Design review of the part shown in the three views and the two pictorial views. Dimensions are in mm from the part's minimum x, y and z. Give positions to 0.01 mm unless a question says otherwise; leave off trailing zeros. Loops run counter-clockwise (first coordinate to the right, second up) from the corner with the lowest first, then second, coordinate; pieces in that order, holes last. Notation, with made-up numbers: (11.5, 88) -> (19.5, 88) arc R22 cw to (19.5, 113) -> close; hole circle Ø4 at (47.5, -13.75). An arc over 180 degrees is marked (long way). Answer as CSV lines item,"result". Start each with the question number.
Item 1: Add section A-A on x = 112.2. State the section outline as (y, z) points, plus the area to 3 significant figures.
Item 2: Add section B-B on z = 23.5. State the section outline as (x, y) points, plus the area to 3 significant figures.
Item 3: Add section D-D on x = 74. State the section outline as (y, z) points, plus the area to 3 significant figures.
Item 4: For L1, parallel to Z at x = 5, y = 1; L2, parallel to X at y = 1.2, z = 71; L3, parallel to X at y = 0.35, z = 37, list the stretches that pass through material, from the lowest coordinate up. Write a range as from..to.
Item 5: Add section C-C on y = 0.5. State how many separate pieces and enclosed holes the cut face has, plus the area to 3 significant figures.
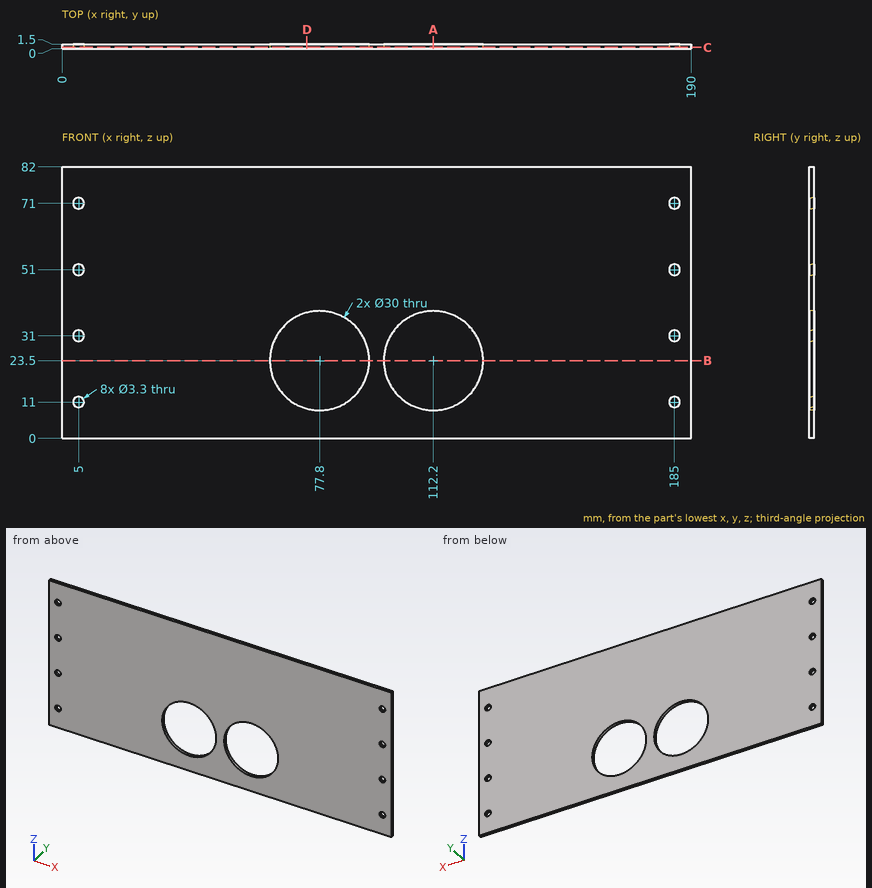
Computed values:
1,outline,"(0, 0) -> (1.5, 0) -> (1.5, 8.5) -> (0, 8.5) -> close; (0, 38.5) -> (1.5, 38.5) -> (1.5, 82) -> (0, 82) -> close"
1,area,"78.0 mm²"
2,outline,"(0, 0) -> (62.8, 0) -> (62.8, 1.5) -> (0, 1.5) -> close; (92.8, 0) -> (97.2, 0) -> (97.2, 1.5) -> (92.8, 1.5) -> close; (127.2, 0) -> (190, 0) -> (190, 1.5) -> (127.2, 1.5) -> close"
2,area,"195 mm²"
3,outline,"(0, 0) -> (1.5, 0) -> (1.5, 8.99) -> (0, 8.99) -> close; (0, 38.01) -> (1.5, 38.01) -> (1.5, 82) -> (0, 82) -> close"
3,area,"79.5 mm²"
4,L1,"0..9.35, 12.65..29.35, 32.65..49.35, 52.65..69.35, 72.65..82"
4,L2,"0..3.35, 6.65..183.35, 186.65..190"
4,L3,"0..71.26, 84.34..105.66, 118.74..190"
5,separate pieces,"1"
5,enclosed holes,"10"
5,area,"14,100 mm²"
